```python
from build123d import *

# Parameters (mm, degrees)
SKETCH_1_W          = 15
SKETCH_1_H          = 15
EXTRUDE_1_DEPTH     = 372
SKETCH_2_R          = 2.6
SKETCH_2_W          = 0.2
SKETCH_2_H          = 0.2
CUT_EXTRUDE_2_DEPTH = 372
SKETCH_3_W          = 370
SKETCH_3_H          = 13
CUT_EXTRUDE_3_DEPTH = 1
SKETCH_4_W          = 15
SKETCH_4_H          = 15
CUT_EXTRUDE_4_DEPTH = 1
SKETCH_5_W          = 15
SKETCH_5_H          = 15
CUT_EXTRUDE_5_DEPTH = 1
SKETCH_6_W          = 12.6
SKETCH_6_H          = 11.399012469
CUT_EXTRUDE_6_DEPTH = 370
SKETCH_7_W          = 15.2
SKETCH_7_H          = 15.1
SKETCH_7_R          = 2.5
EXTRUDE_4_DEPTH     = 1
EXTRUDE_START       = 1
SKETCH_8_W          = 15.2
SKETCH_8_H          = 15.1
SKETCH_8_R          = 2.5
EXTRUDE_5_DEPTH     = 1


with BuildPart() as part:
    # 草图1 → 凸台-拉伸1 (new body)
    with BuildSketch(Plane(origin=(0, 0, 0), x_dir=(0, 0, -1), z_dir=(1, 0, 0))):
        with Locations((-16.757142857, 9.442767842)):
            Rectangle(SKETCH_1_W, SKETCH_1_H)
    extrude(amount=EXTRUDE_1_DEPTH)

    # 草图2 → 切除-拉伸2 (cut)
    with BuildSketch(Plane(origin=(372, 0, 0), x_dir=(0, 0, -1), z_dir=(1, 0, 0))):
        with Locations((-16.757142857, 9.442767842)):
            Circle(SKETCH_2_R)
        with Locations((-24.157142857, 15.588150761)):
            Rectangle(SKETCH_2_W, SKETCH_2_H)
        with Locations((-9.357142857, 15.588150761)):
            Rectangle(SKETCH_2_W, SKETCH_2_H)
    extrude(amount=-CUT_EXTRUDE_2_DEPTH, mode=Mode.SUBTRACT)

    # 草图3 → 切除-拉伸3 (cut)
    with BuildSketch(Plane.XZ.offset(-1.942767842)):
        with Locations((186, 16.757142857)):
            Rectangle(SKETCH_3_W, SKETCH_3_H)
    extrude(amount=-CUT_EXTRUDE_3_DEPTH, mode=Mode.SUBTRACT)

    # 草图4 → 切除-拉伸4 (cut)
    with BuildSketch(Plane.ZY):
        with Locations((16.757142857, 9.442767842)):
            Rectangle(SKETCH_4_W, SKETCH_4_H)
    extrude(amount=-CUT_EXTRUDE_4_DEPTH, mode=Mode.SUBTRACT)

    # 草图5 → 切除-拉伸5 (cut)
    with BuildSketch(Plane(origin=(372, 0, 0), x_dir=(0, 0, -1), z_dir=(1, 0, 0))):
        with Locations((-16.757142857, 9.442767842)):
            Rectangle(SKETCH_5_W, SKETCH_5_H)
    extrude(amount=-CUT_EXTRUDE_5_DEPTH, mode=Mode.SUBTRACT)

    # 草图6 → 切除-拉伸6 (cut)
    with BuildSketch(Plane(origin=(371, 0, 0), x_dir=(0, 0, -1), z_dir=(1, 0, 0))):
        with Locations((-16.757142857, 9.243261608)):
            Rectangle(SKETCH_6_W, SKETCH_6_H)
    extrude(amount=-CUT_EXTRUDE_6_DEPTH, mode=Mode.SUBTRACT)

    # 草图7 → 凸台-拉伸4 (add)
    with BuildSketch(Plane(origin=(371, 0, 0), x_dir=(0, 0, -1), z_dir=(1, 0, 0))):
        with Locations((-16.757142857, 9.392767842)):
            Rectangle(SKETCH_7_W, SKETCH_7_H)
        with Locations((-16.757142857, 9.392767842)):
            Circle(SKETCH_7_R, mode=Mode.SUBTRACT)
    extrude(amount=EXTRUDE_4_DEPTH)

    # 草图8 → 凸台-拉伸5 (add)
    with BuildSketch(Plane.ZY.offset(-1).offset(EXTRUDE_START)):
        with Locations((16.757142857, 9.392767842)):
            Rectangle(SKETCH_8_W, SKETCH_8_H)
        with Locations(Location((16.757142857, 9.392767842, 0), (0, 0, 180))):
            Circle(SKETCH_8_R, mode=Mode.SUBTRACT)
    extrude(amount=-EXTRUDE_5_DEPTH)


solid = part.part
```
Verification items for the finished model (mm, model axes). A direction names the side the tool comes from. Round coordinates to 2 decimals unless told otherwise and drop trailing zeros. Write each loop counter-clockwise with the first axis right and the second up, starting at its lowest first coordinate (ties: lowest second). Pieces come first, ordered by that corner, then holes.
1. Gauge pin test, flat ends, axial feed: P1, Ø0.5, axis at x = 124.5, z = 10, coming from the -Y side; P2, Ø1.1, axis at x = 167, y = 2.5, coming from the +Z side; P3, Ø4, axis at x = 272.5, z = 18, coming from the -Y side. Record the tip position at first contact, or that the pin passes through.
2. Draft check along Z on faces 4 (the flat face through (183, 9, 9.257)), 5 (the flat face through (183, 16.943, 17)), 6 (the flat face through (1, 9, 14)), 7 (the flat face through (371, 9, 20)). Enter one of: +Z half, -Z half, draft (parallel to the pull), parting line (faces both ways), or undercut.
3. Scan lines: L1, parallel to X at y = 13.75, z = 19.5; L2, parallel to Y at x = 212, z = 10.5; L3, parallel to Z at x = 192, y = 3.75. Record each from-to range of solid material in increasing order.
4. Access from +Z, -Z, +X, -X, +Y, -Y to the whole of each face (thin tool, end or side, straight path). Record for faces 1 (the flat face through (372, 11, 19)), 2 (the flat face through (189, 3.544, 17)), 3 (the flat face through (183, 2.943, 17)).
5. Section check A-A on x = 340.5. Enter the section's corners in (y, z), plus the area to 3 significant figures.
Answer:
1. P1: stops at y = 1.94
1. P2: stops at z = 24.26
1. P3: stops at y = 2.94
2. face 4: -Z half
2. face 5: draft
2. face 6: undercut
2. face 7: undercut
3. L1: x = 0 to 1, 371 to 372
3. L2: y = 2.94 to 3.54, 14.94 to 16.94
3. L3: z = 9.26 to 10.46, 23.06 to 24.26
4. face 1: +Z, -Z, +X, +Y, -Y
4. face 2: none
4. face 3: -Y
5. outline: (1.94, 9.26) - (15.49, 9.26) - (15.49, 9.46) - (15.69, 9.46) - (15.69, 9.26) - (16.94, 9.26) - (16.94, 24.26) - (15.69, 24.26) - (15.69, 24.06) - (15.49, 24.06) - (15.49, 24.26) - (1.94, 24.26) - (1.94, 23.26) - (2.94, 23.26) - (2.94, 10.26) - (1.94, 10.26) - close; hole (3.54, 10.46) - (14.94, 10.46) - (14.94, 23.06) - (3.54, 23.06) - close
5. area: 68.3 mm2
